Model file for the job. Use its own axes, mm. Face numbers are marked on the shaded views. Coordinates: 2 decimals unless noted, no trailing zeros. Order: outer loops, then holes, each group sorted by start corner. A loop starts at its lowest first (then second) coordinate and runs counter-clockwise, first axis right, second up.
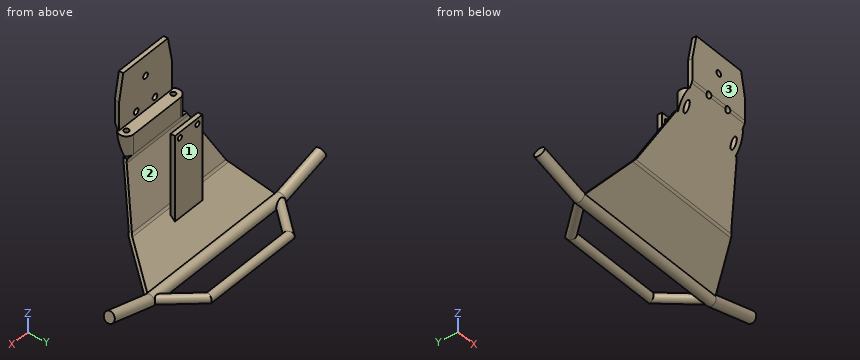
from build123d import *

# Parameters (mm, degrees)
BOSS_EXTRUDE1_DEPTH             = 57
SKETCH18_R                      = 2
CUT_EXTRUDE3_DEPTH              = 3
CUT_EXTRUDE5_DEPTH              = 60
CUT_EXTRUDE5_DEPTH_BACK         = 1.0000001
SKETCH24_R                      = 1.7
CUT_EXTRUDE6_DEPTH              = 14
SWEEP1_PROFILE_R                = 3.75
SWEEP2_PROFILE_R                = 3
BOSS_EXTRUDE2_REACH             = 77.667
SKETCH19_W                      = 23.25
SKETCH19_H                      = 3
BOSS_EXTRUDE2_DIRECTION_2_DEPTH = 5
CUT_EXTRUDE8_REACH              = 35
SKETCH54_R                      = 1.75


with BuildPart() as part:
    # Sketch2 → Boss-Extrude1 (new body, symmetric)
    with BuildSketch(Plane(origin=(0, 0, 0), x_dir=(0, 0, -1), z_dir=(1, 0, 0))):
        with BuildLine():
            Line((0, 0), (32.709545462, 0))
            ThreePointArc((32.709545462, 0), (33.775734101, 0.114998282), (34.792878796, 0.454703286))
            Line((34.792878796, 0.454703286), (87.43170835, 24.581671255))
            ThreePointArc((87.43170835, 24.581671255), (88.285761732, 25.080764899), (89.024845605, 25.738227198))
            Line((89.024845605, 25.738227198), (111.387831165, 50))
            Line((111.387831165, 50), (109.917242929, 51.355496308))
            Line((109.917242929, 51.355496308), (87.826438044, 27.389014385))
            ThreePointArc((87.826438044, 27.389014385), (87.087354171, 26.731552087), (86.233300789, 26.232458442))
            Line((86.233300789, 26.232458442), (53.992045448, 11.454703286))
            ThreePointArc((53.992045448, 11.454703286), (52.974900754, 11.114998282), (51.908712115, 11))
            Line((51.908712115, 11), (38, 11))
            Line((38, 11), (38, 3))
            Line((38, 3), (0, 3))
            Line((0, 3), (0, 0))
        make_face()
    extrude(amount=BOSS_EXTRUDE1_DEPTH, both=True)

    # Sketch18 → Cut-Extrude3 (cut)
    with BuildSketch(Plane(origin=(0, 3, 0), x_dir=(1, 0, 0), z_dir=(0, 1, 0))):
        with Locations((-8, 34)):
            Circle(SKETCH18_R)
        with Locations((8, 34)):
            Circle(SKETCH18_R)
        with Locations((0, 14)):
            Circle(SKETCH18_R)
    extrude(amount=-CUT_EXTRUDE3_DEPTH, mode=Mode.SUBTRACT)

    # Sketch23 → Cut-Extrude5 (cut, two sides)
    with BuildSketch(Plane(origin=(0, 0, 0), x_dir=(1, 0, 0), z_dir=(0, 1, 0))) as cut_extrude5_sk:
        Polygon((19, 0), (22.5, 18), (22.5, 38), (25.5, 38), (25.5, 51.908712115), (40, 86.233300789), (57, 111.387831165), (57, 0), align=None)
        Polygon((-57, 0), (-19, 0), (-22.5, 18), (-22.5, 38), (-25.5, 38), (-25.5, 51.908712115), (-40, 86.233300789), (-57, 111.387831165), align=None)
    extrude(amount=CUT_EXTRUDE5_DEPTH, mode=Mode.SUBTRACT)
    extrude(cut_extrude5_sk.sketch, amount=-CUT_EXTRUDE5_DEPTH_BACK, mode=Mode.SUBTRACT)

    # Sketch24 → Cut-Extrude6 (cut)
    with BuildSketch(Plane.XY.offset(-38)):
        with Locations((-20, 6)):
            Circle(SKETCH24_R)
        with Locations((20, 6)):
            Circle(SKETCH24_R)
        with BuildLine():
            Line((-20, 11), (-25.5, 11))
            Line((-25.5, 11), (-25.5, 1.924684879))
            Line((-25.5, 1.924684879), (-22.89686152, 1.924684879))
            ThreePointArc((-22.89686152, 1.924684879), (-24.763222418, 7.520431583), (-20, 11))
        make_face()
        with BuildLine():
            Line((22.89686152, 1.924684879), (25.5, 1.924684879))
            Line((25.5, 1.924684879), (25.5, 11))
            Line((25.5, 11), (20, 11))
            ThreePointArc((20, 11), (24.763222418, 7.520431583), (22.89686152, 1.924684879))
        make_face()
    extrude(amount=-CUT_EXTRUDE6_DEPTH, mode=Mode.SUBTRACT)

    # Sweep1: sweep along a curve in space
    with BuildLine() as sweep1_path:
        Line((-90, 51.35, -100), (-56.006143242, 51.355496308, -109.917242929))
        Line((-56.006143242, 51.355496308, -109.917242929), (56.006143242, 51.355496308, -109.917242929))
        Line((56.006143242, 51.355496308, -109.917242929), (90, 51.35, -100))
    # Sweep1 profile (on start of the path) → Sweep1 (sweep)
    with BuildSketch(Plane(origin=(-90, 51.35, -100), x_dir=(0.28006163, 0, 0.959982023), z_dir=(0.959982011, 0.000155215, -0.280061626))):
        Circle(SWEEP1_PROFILE_R)
    sweep(path=sweep1_path.line, transition=Transition.RIGHT)

    # Sweep2: sweep along a curve in space
    with BuildLine() as sweep2_path:
        Line((-56, 50, -110), (-34, 75, -110))
        Line((-34, 75, -110), (34, 75, -110))
        Line((34, 75, -110), (56, 50, -110))
    # Sweep2 profile (on start of the path) → Sweep2 (sweep)
    with BuildSketch(Plane(origin=(-56, 50, -110), x_dir=(0.750713517, -0.660627895, 0), z_dir=(0.660627895, 0.750713517, 0))):
        Circle(SWEEP2_PROFILE_R)
    sweep(path=sweep2_path.line, transition=Transition.RIGHT)

    # Boss-Extrude2: up to this face of the body (flat: up to its plane)
    boss_extrude2_end = Plane(part.part.faces().sort_by_distance((0, 38.483295154, -98.05245255))[0])
    # Sketch19 → Boss-Extrude2 (add, up to the picked face)
    with BuildSketch(Plane.XY.offset(-38), mode=Mode.PRIVATE) as boss_extrude2_sk1:
        with Locations((0, 31.5)):
            Rectangle(SKETCH19_W, SKETCH19_H)
    boss_extrude2_tool1 = split(extrude(boss_extrude2_sk1.sketch, amount=-BOSS_EXTRUDE2_REACH, mode=Mode.PRIVATE), bisect_by=boss_extrude2_end, keep=Keep.BOTH, mode=Mode.PRIVATE)
    add(boss_extrude2_tool1.solids().sort_by_distance((0, 31.5, -38))[0])

    # Sketch19 → Boss-Extrude2 direction 2 (add)
    with BuildSketch(Plane.XY.offset(-38)):
        with Locations((0, 31.5)):
            Rectangle(SKETCH19_W, SKETCH19_H)
    extrude(amount=BOSS_EXTRUDE2_DIRECTION_2_DEPTH)

    # Sketch54 → Cut-Extrude8 (cut, up to next)
    with BuildSketch(Plane(origin=(0, 33, 0), x_dir=(1, 0, 0), z_dir=(0, 1, 0)), mode=Mode.PRIVATE) as cut_extrude8_sk1:
        with Locations((-7.5, 37)):
            Circle(SKETCH54_R)
    cut_extrude8_tool1 = extrude(cut_extrude8_sk1.sketch, amount=-CUT_EXTRUDE8_REACH, mode=Mode.PRIVATE) & part.part
    add(cut_extrude8_tool1.solids().sort_by_distance((-7.5, 33, -37))[0], mode=Mode.SUBTRACT)
    # Sketch54 → Cut-Extrude8 (cut, up to next)
    with BuildSketch(Plane(origin=(0, 33, 0), x_dir=(1, 0, 0), z_dir=(0, 1, 0)), mode=Mode.PRIVATE) as cut_extrude8_sk2:
        with Locations((7.5, 37)):
            Circle(SKETCH54_R)
    cut_extrude8_tool2 = extrude(cut_extrude8_sk2.sketch, amount=-CUT_EXTRUDE8_REACH, mode=Mode.PRIVATE) & part.part
    add(cut_extrude8_tool2.solids().sort_by_distance((7.5, 33, -37))[0], mode=Mode.SUBTRACT)


solid = part.part
Q1. Drop flat-ended pins along their axis: P1, Ø0.9, axis at y = 31, z = -51.5, coming from the -X side (3 decimals); P2, Ø10, axis at x = 1.5, z = -30, coming from the +Y side; P3, Ø3.5, axis at x = 5.5, y = 31, coming from the +Z side. Give the stop position or say it passes through.
Established:
P1: stops at x = -11.625
P2: stops at y = 33
P3: stops at z = -33
Q2. Cut at C-C, the plane z = -73. List the corners of the cut face in (x, y) (3 decimals), plus the area to 3 significant figures.
Established:
outline: (-34.41, 17.967) - (34.41, 17.967) - (34.41, 20.167) - (-34.41, 20.167) - close; (-11.625, 30) - (11.625, 30) - (11.625, 33) - (-11.625, 33) - close
area: 221 mm2
Q3. Cut at A-A, the plane x = 0. List the corners of the cut face in (y, z).
Established:
outline: (0, -32.71) arc R5 ccw to (0.45, -34.79) - (24.58, -87.43) arc R5 ccw to (25.74, -89.02) - (47.67, -109.24) arc R3.75 ccw (long way) to (48.6, -107.38) - (33, -93) - (33, -33) - (30, -33) - (30, -90.23) - (27.39, -87.83) arc R5 cw to (26.23, -86.23) - (11.45, -53.99) arc R5 cw to (11, -51.91) - (11, -38) - (3, -38) - (3, -16) - (0, -16) - close; (0, -12) - (3, -12) - (3, 0) - (0, 0) - close; circle Ø6 at (75, -110)
Q4. Probe line 1 (X direction, y = 6, z = -42); line 2 (X direction, y = 31.2, z = -37) (3 decimals); line 3 (X direction, y = 1.75, z = -14). List the from-to ranges inside material, lowest first.
Established:
line 1: x = -25 to -21.7, -18.3 to 18.3, 21.7 to 25
line 2: x = -11.625 to -9.25, -5.75 to 5.75, 9.25 to 11.625
line 3: x = -21.72 to -2, 2 to 21.72
Q5. Cut at D-D, the plane y = 19. List the corners of the cut face in (x, z), plus the area to 3 significant figures.
Established:
outline: (-35.36, -75.25) - (35.36, -75.25) - (33.33, -70.45) - (-33.33, -70.45) - close
area: 330 mm2
Q6. Mould opens along Y. For the marked faces 1, 2 and 3 say: pulls with the +Y half, pulls with the -Y half, needs draft (parallel to the pull), parting line crosses it, or undercut.
Established:
face 1: pulls with the +Y half
face 2: undercut
face 3: pulls with the -Y half
Q7. Cut at B-B, the plane z = -14. List the corners of the cut face in (x, y).
Established:
outline: (-21.72, 0) - (-2, 0) - (-2, 3) - (-21.72, 3) - close; (2, 0) - (21.72, 0) - (21.72, 3) - (2, 3) - close
